Read the model definition and answer for the solid it produces. Units are mm, in the model's axes. A direction names the side the tool comes from. Round coordinates to 2 decimals unless told otherwise and drop trailing zeros. Loops run counter-clockwise (first coordinate to the right, second up) from the corner with the lowest first, then second, coordinate; pieces in that order, holes last. Notation, with made-up numbers: (75.25, 70) - (93.25, 70) arc R24 cw to (93.25, 104) - close; hole circle Ø11 at (26.25, 5). An arc over 180 degrees is marked (long way). Use CSV: the item, a comma, the result in double quotes. Start each with the question number.
1. A tool of negligible diameter and unlimited length cuts with its end or side. For faces 1 (the flat face through (10, 51, 0)), 2 (the flat face through (10, 49, 2)), from which of +Z, -Z, +X, -X, +Y, -Y can it reach the whole face along a straight path? Write none if from no direction.
2. Consider line 1 along X through (y, z) = (53, 14.25); line 2 along X through (y, z) = (86, 19.25). Determine where each line is inside the solid, lowest interval first.
3. Find section A-A (z = 17). Give the vertices of the cut face in (x, y).
4. Find section B-B (y = 14.5). Give the vertices of the cut face in (x, z), and give its area (3 significant figures).
5. Find section C-C (x = 10.5). Give the vertices of the cut face in (y, z), and give its area (3 significant figures).
6. Determine the mould class of faces 3 (the flat face through (10, 49, 18)), 4 (the flat face through (10, 0, 19)), 5 (the flat face through (0, 49, 10)) for opening direction X: +X half, -X half, draft (parallel to the pull), parting line (faces both ways), or undercut.
from build123d import *

# Parameters (mm, degrees)
SKETCH_W     = 20
SKETCH_H     = 100
PAD_DEPTH    = 20
SKETCH001_W  = 16
SKETCH001_H  = 16
POCKET_DEPTH = 100.001
FILLET_R     = 1
FILLET001_R  = 1
FILLET002_R  = 1


with BuildPart() as part:
    # Sketch → Pad (new body)
    with BuildSketch(Plane.XY):
        with Locations((10, 50)):
            Rectangle(SKETCH_W, SKETCH_H)
    extrude(amount=PAD_DEPTH)

    # Sketch001 (on Face1 of Pad) → Pocket (cut, through all)
    with BuildSketch(Plane.XZ):
        with Locations((10, 10)):
            Rectangle(SKETCH001_W, SKETCH001_H)
    extrude(amount=-POCKET_DEPTH, mode=Mode.SUBTRACT)

    # Fillet
    fillet_edges = [part.edges().sort_by_distance(p)[0] for p in [
        (20, 50, 20),
    ]]
    fillet(fillet_edges, radius=FILLET_R)

    # Fillet001
    fillet001_edges = [part.edges().sort_by_distance(p)[0] for p in [
        (0, 50, 20),
    ]]
    fillet(fillet001_edges, radius=FILLET001_R)

    # Fillet002
    fillet002_edges = [part.edges().sort_by_distance(p)[0] for p in [
        (0, 50, 0),
        (20, 50, 0),
    ]]
    fillet(fillet002_edges, radius=FILLET002_R)


solid = part.part
Filled sheet:
1,face 1,"-Z, +X, -X, +Y, -Y"
1,face 2,"+Y, -Y"
2,line 1,"x = 0 to 2, 18 to 20"
2,line 2,"x = 0.03 to 19.97"
3,outline,"(0, 0) - (2, 0) - (2, 100) - (0, 100) - close; (18, 0) - (20, 0) - (20, 100) - (18, 100) - close"
4,outline,"(0, 1) arc R1 ccw to (1, 0) - (19, 0) arc R1 ccw to (20, 1) - (20, 19) arc R1 ccw to (19, 20) - (1, 20) arc R1 ccw to (0, 19) - close; hole (2, 2) - (18, 2) - (18, 18) - (2, 18) - close"
4,area,"143 mm²"
5,outline,"(0, 0) - (100, 0) - (100, 2) - (0, 2) - close; (0, 18) - (100, 18) - (100, 20) - (0, 20) - close"
5,area,"400 mm²"
6,face 3,"undercut"
6,face 4,"draft"
6,face 5,"-X half"
